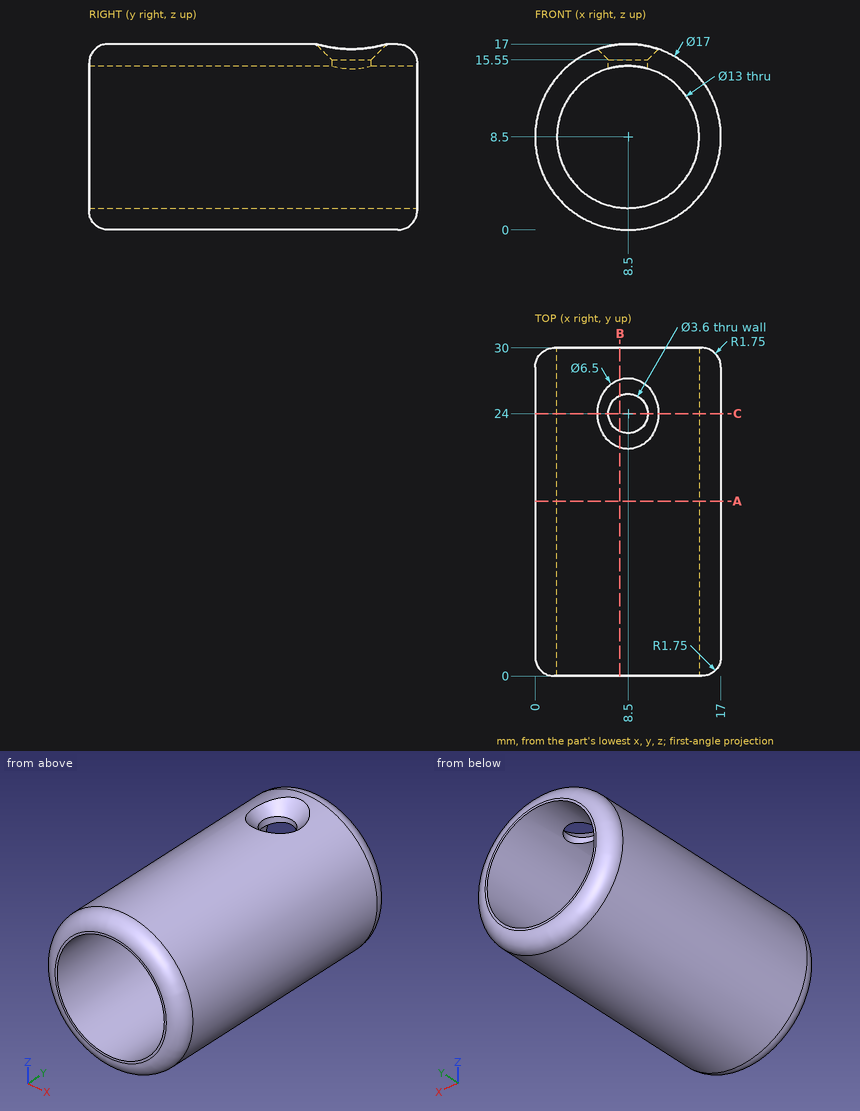
Study the drawing (mm; zero at the part's minimum x, y, z) and answer. Give positions to 0.01 mm unless a question says otherwise; leave off trailing zeros. Write each loop counter-clockwise with the first axis right and the second up, starting at its lowest first coordinate (ties: lowest second). Pieces come first, ordered by that corner, then holes. Notation, with made-up numbers: (-39.75, 4.5) -> (-3.75, 4.5) arc R32 ccw to (-3.75, 36.5) -> close; hole circle Ø11 at (32, 77). An arc over 180 degrees is marked (long way). Answer in a Markdown table with one row per item.
1) Section C-C on y = 24 is taken. Give the vertices of the cut face in (x, z), plus the area to 3 significant figures.
Results list:
| item | result |
|---|---|
| outline | (5.72, 16.53) arc R8.5 ccw (long way) to (11.28, 16.53) -> (10.3, 15.55) -> (10.3, 14.75) arc R6.5 cw (long way) to (6.7, 14.75) -> (6.7, 15.55) -> close |
| area | 85.7 mm^2 |
2) Section A-A on y = 16 is taken. Give the vertices of the cut face in (x, z), plus the area to 3 significant figures.
Results list:
| item | result |
|---|---|
| outline | circle Ø17 at (8.5, 8.5); hole circle Ø13 at (8.5, 8.5) |
| area | 94.2 mm^2 |
3) Straight lines are drawn through the part: line 1 (Z direction, x = 8.5, y = 12); line 2 (Z direction, x = 6.75, y = 19.5); line 3 (X direction, y = 28, z = 2.5). For each, find the intervals that lie inside material, in ascending order. Write a range as [from, to].
Results list:
| item | result |
|---|---|
| line 1 | [0, 2], [15, 17] |
| line 2 | [0.18, 2.24], [14.76, 16.82] |
| line 3 | [2.48, 6], [11, 14.52] |
4) Section B-B on x = 7.75 is taken. Count the separate pieces of the cut face and the enclosed holes in it, plus the area to 3 significant figures.
Results list:
| item | result |
|---|---|
| separate pieces | 3 |
| enclosed holes | 0 |
| area | 109 mm^2 |
5) Each of these flat-tipped pins is pushed along its axis until it touches: pin 1 Ø4 at (x, y) = (14, 25) entering from -Z; pin 2 Ø2 at (x, y) = (11, 18.5) entering from -Z; pin 3 Ø4 at (y, z) = (22, 3) entering from -X. Where does it stop, or does it pass through?
Results list:
| item | result |
|---|---|
| pin 1 | z = 0.75 |
| pin 2 | z = 0.13 |
| pin 3 | x = 0.75 |
